Source: CAD feature listing. Evaluate the final solid. Frame: model axes, mm. A direction names the side the tool comes from. Round coordinates to 2 decimals unless told otherwise and drop trailing zeros. Write each loop counter-clockwise with the first axis right and the second up, starting at its lowest first coordinate (ties: lowest second). Pieces come first, ordered by that corner, then holes. Notation, with made-up numbers: M 36.5,-11 L 92.5,-11 A17 ccw 92.5,-4 Z; hole C -36.75,-28.75 d11. An arc over 180 degrees is marked long. Answer in a Markdown table with one row per item. Add a question column.
Item 1: Mould query, pull axis Z, two halves, no side actions, for faces 4 (the face through (0, 5.334, 0)), 5 (the face through (1.53, 0.63, -3.04)), 6 (the face through (1.2, 6.35, 1.3)), 7 (the face through (0, 3.8, 3.1)). Classes: released by +Z, released by -Z, zero draft, split by the parting line, or undercut.
Item 2: Material intervals for probe 1 along X at (y, z) = (5.65, 0); probe 2 along X at (y, z) = (1.25, 0); probe 3 along Y at (x, z) = (1.75, 4.5), sorted ascending.
Item 3: Cut plane D-D on y = 3.75. Return loops of the section in (x, z), and give its area (3 significant figures).
Item 4: Contact query for flat-ended pins moving along their axis: pin 1 (2 mm diameter, centred on x = -1, y = 4.5, fed in from +Z); pin 2 (0.6 mm diameter, centred on x = 0, z = -3.5, fed in from +Y); pin 3 (1.3 mm diameter, centred on x = -0.5, z = 0, fed in from +Y). Output: stop coordinate, or through.
Item 5: Set-up query: faces 1 (the face through (0, 3.8, -3.1)), 2 (the face through (-2.604, 3, 0)), 3 (the face through (3, 0, 0)). Return all of +Z, -Z, +X, -X, +Y, -Y with unobstructed straight access to the full face (end or side cutting, diameter ignored); none if empty.
Item 6: Cut plane C-C on x = 0. Return loops of the section in (y, z).
Item 7: Cut plane B-B on y = 0.5. Return loops of the section in (x, z), and give its area (3 significant figures).
Autodesk Inventor part; units mm, degrees
ref_plane "body_XY" through (0, -0.762, 0) normal (0, 1, 0) x (1, 0, 0)
ref_plane "body_YZ" through (0, -0.762, 0) normal (1, 0, 0) x (0, 0, -1)
ref_plane "body_ZX" through (0, -0.762, 0) normal (0, 0, -1) x (0, 1, 0)
sketch "Sketch_1" plane through (0, 0, 0) normal (0, 1, 0) x (-1, 0, 0)
  line L0 (3.302, -6.223) -> (3.302, 6.223)
  arc A0 (3.302, 6.223) -> (3.175, 6.35) centre (3.175, 6.223) ccw
  line L1 (3.175, 6.35) -> (-3.175, 6.35)
  arc A1 (-3.175, 6.35) -> (-3.302, 6.223) centre (-3.175, 6.223) ccw
  line L2 (-3.302, 6.223) -> (-3.302, -6.223)
  arc A2 (-3.302, -6.223) -> (-3.175, -6.35) centre (-3.175, -6.223) ccw
  line L3 (-3.175, -6.35) -> (3.175, -6.35)
  arc A3 (3.175, -6.35) -> (3.302, -6.223) centre (3.175, -6.223) ccw
extrude "Extrusion1" add sketch "Sketch_1" against normal blind 0.762
sketch "Sketch_2" plane through (0, 0, 0) normal (0, 0, 1) x (1, 0, 0)
  line L0 (-3.302, 0.254) -> (-3.302, -0.127)
  arc A0 (-3.175, 0) -> (-3.302, -0.127) centre (-3.175, -0.127) ccw
  line L1 (-3.175, 0) -> (3.175, 0)
  arc A1 (3.302, -0.127) -> (3.175, 0) centre (3.175, -0.127) ccw
  line L2 (3.302, -0.127) -> (3.302, 0.254)
  line L3 (3.302, 0.254) -> (-3.302, 0.254)
extrude "Extrusion2" cut sketch "Sketch_2" along normal mid plane 12.7
sketch "Sketch_3" plane through (0, 0, 0) normal (1, 0, 0) x (0, 1, 0)
  line L0 (0.254, 6.35) -> (-0.127, 6.35)
  arc A0 (0, 6.223) -> (-0.127, 6.35) centre (-0.127, 6.223) ccw
  line L1 (0, 6.223) -> (0, -6.223)
  arc A1 (-0.127, -6.35) -> (0, -6.223) centre (-0.127, -6.223) ccw
  line L2 (-0.127, -6.35) -> (0.254, -6.35)
  line L3 (0.254, -6.35) -> (0.254, 6.35)
extrude "Extrusion3" cut sketch "Sketch_3" along normal mid plane 12.7
sketch "Sketch_4" plane through (0, 0, 0) normal (1, 0, 0) x (0, 1, 0)
  line L0 (0, 0) -> (6.35, 0)
  line L1 (5.334, 0) -> (5.334, -1.27)
  line L2 (5.334, -1.27) -> (6.223, -1.27)
  arc A0 (6.35, -1.397) -> (6.223, -1.27) centre (6.223, -1.397) ccw
  line L3 (6.35, -1.397) -> (6.35, -2.8448)
  arc A1 (6.096, -3.0988) -> (6.35, -2.8448) centre (6.096, -2.8448) ccw
  line L4 (6.096, -3.0988) -> (1.524, -3.0988)
  line L5 (1.524, -3.0988) -> (1.27, -3.4036)
  line L6 (1.27, -3.4036) -> (0, -3.4036)
  line L7 (0, -3.4036) -> (0, 0)
  line L8 (0, 0) -> (5.334, 0)
revolve "Revolution1" add sketch "Sketch_4" angle 360 about axis through (0, 0, 0) along (0, -1, 0)
sketch "Sketch_5" plane through (0, 0, 0) normal (0, 1, 0) x (-1, 0, 0)
  line L0 (0.254, -3.6068) -> (0.254, 3.6068)
  arc A0 (0.254, 3.6068) -> (-0.254, 3.6068) centre (0, 3.6068) ccw
  line L1 (-0.254, 3.6068) -> (-0.254, -3.6068)
  arc A1 (-0.254, -3.6068) -> (0.254, -3.6068) centre (0, -3.6068) ccw
extrude "Extrusion4" add sketch "Sketch_5" along normal blind 1.524
sketch "Sketch_6" plane through (0, 6.35, 0) normal (0, 1, 0) x (1, 0, 0)
  line L0 (-3.8735, -5.08) -> (3.8735, -5.08)
  line L1 (3.8735, -5.08) -> (3.8735, 5.08)
  line L2 (3.8735, 5.08) -> (-3.8735, 5.08)
  line L3 (-3.8735, 5.08) -> (-3.8735, -5.08)
  line L4 (-2.6035, 4.572) -> (-2.6035, -4.572)
  line L5 (-2.6035, -4.572) -> (2.6035, -4.572)
  line L6 (2.6035, -4.572) -> (2.6035, 4.572)
  line L7 (2.6035, 4.572) -> (-2.6035, 4.572)
extrude "Extrusion5" cut sketch "Sketch_6" against normal blind 6.35
ref_plane "body_XY" through (0, -0.762, 0) normal (0, 1, 0) x (1, 0, 0)
ref_plane "body_YZ" through (0, -0.762, 0) normal (1, 0, 0) x (0, 0, -1)
ref_plane "body_ZX" through (0, -0.762, 0) normal (0, 0, -1) x (0, 1, 0)
ref_plane "bus_brac_XY" through (0, 0, 0) normal (0, -1, 0) x (1, 0, 0)
ref_plane "bus_brac_YZ" through (0, 0, 0) normal (1, 0, 0) x (0, 0, 1)
ref_plane "bus_brac_ZX" through (0, 0, 0) normal (0, 0, 1) x (0, -1, 0)
ref_plane "toggle_XY" through (0, 6.35, 0) normal (0, -1, 0) x (1, 0, 0)
ref_plane "toggle_YZ" through (0, 6.35, 0) normal (1, 0, 0) x (0, 0, 1)
ref_plane "toggle_ZX" through (0, 6.35, 0) normal (0, 0, 1) x (0, -1, 0)
properties part number "M2T12A5bush"
Results below:
| question | item | result |
|---|---|---|
| 1 | face 4 | undercut |
| 1 | face 5 | released by -Z |
| 1 | face 6 | zero draft |
| 1 | face 7 | released by +Z |
| 2 | probe 1 | -2.6 to -1.27, 1.27 to 2.6 |
| 2 | probe 2 | -2.6 to 2.6 |
| 2 | probe 3 | -0.76 to 0 |
| 3 | outline | M -2.6,-1.68 A3.1 ccw 2.6,-1.68 L 2.6,1.68 A3.1 ccw -2.6,1.68 Z |
| 3 | area | 27.9 mm2 |
| 4 | pin 1 | z = 3.1 |
| 4 | pin 2 | y = 1.52 |
| 4 | pin 3 | y = 5.33 |
| 5 | face 1 | -Z, +Y |
| 5 | face 2 | +Z, -Z, -X, +Y |
| 5 | face 3 | +Y |
| 6 | outline | M -0.76,-6.35 L -0.13,-6.35 A0.13 ccw 0,-6.22 L 0,-3.86 L 1.52,-3.86 L 1.52,-3.1 L 6.1,-3.1 A0.25 ccw 6.35,-2.84 L 6.35,-1.4 A0.13 ccw 6.22,-1.27 L 5.33,-1.27 L 5.33,1.27 L 6.22,1.27 A0.13 ccw 6.35,1.4 L 6.35,2.84 A0.25 ccw 6.1,3.1 L 1.52,3.1 L 1.52,3.86 L 0,3.86 L 0,6.22 A0.13 ccw -0.13,6.35 L -0.76,6.35 Z |
| 7 | outline | M -2.6,-2.19 A3.4 ccw -0.25,-3.39 L -0.25,-3.61 A0.25 ccw 0.25,-3.61 L 0.25,-3.39 A3.4 ccw 2.6,-2.19 L 2.6,2.19 A3.4 ccw 0.25,3.39 L 0.25,3.61 A0.25 ccw -0.25,3.61 L -0.25,3.39 A3.4 ccw -2.6,2.19 Z |
| 7 | area | 32.0 mm2 |
